CAD build for the part. Positions are in the model's coordinates, mm. A direction names the side the tool comes from. Give positions to 0.01 mm unless a question says otherwise; leave off trailing zeros. Order: outer loops, then holes, each group sorted by start corner. A loop starts at its lowest first (then second) coordinate and runs counter-clockwise, first axis right, second up. Notation, with made-up numbers: (5.5, 7.25) -> (32.5, 7.25) arc R15 ccw to (32.5, 36.25) -> close; hole circle Ø11 at (57, -15). An arc over 180 degrees is marked (long way). Use one line per item in the form item = value. Start each with the question number.
1) Tool access for faces 4 (the face through (0, 0, -6)), 5 (the face through (0.86, 0.51, 1.06)): list every direction of +Z, -Z, +X, -X, +Y, -Y with a clear straight run to the whole face (end or side of a thin tool).
2) Probe line 1 (Y direction, x = -0.55, z = 1.25); line 2 (Y direction, x = 0.4, z = 0.5); line 3 (Y direction, x = -0.2, z = -5.5). List the from-to ranges inside material, lowest first.
3) Cut at A-A, the plane z = -1. Give the cut face in (x, y), and give its area (3 significant figures).
4) Drop flat-ended pins along their axis: P1, Ø0.5, axis at x = 0, z = 1, coming from the -Y side; P2, Ø3, axis at y = -1.5, z = -3, coming from the +X side; P3, Ø3, axis at y = -1.5, z = -3, coming from the -X side. Give the stop position or say it passes through.
5) Mould opens along X. For faces 1 (the face through (0.1, 0, 0)), 2 (the face through (0, 2, 0)), 3 (the face through (-1.5, 0.07, -2.87)) say: pulls with the +X half, pulls with the -X half, needs draft (parallel to the pull), parting line crosses it, or undercut.
Solid Edge part; units mm, degrees
sketch "Sketch1" plane through (0, 0, 0) normal (0, -1, 0) x (1, 0, 0)
  line L0 (0, -6) -> (1.5, -6)
  line L1 (1.5, -6) -> (1.5, -0.115)
  arc A0 (1.5, -0.105) -> (1.5, -0.115) centre (1.5038, -0.11) ccw
  line L2 (1.5, -0.105) -> (1.5, 0)
  line L3 (1.5, 0) -> (2.85, 0)
  line L4 (2.85, 0) -> (2.85, 0.165)
  arc A1 (1.27, 1.65) -> (2.85, 0.165) centre (-0.3628, -1.6703) cw
  line L5 (0, 1.65) -> (1.27, 1.65)
  dimension "D1" = 1.5
revolve "RevolvedProtrusion1" add sketch "Sketch1" angle 360 about axis through (0, 0, 5) along (0, 0, -1)
sketch "Sketch2" plane through (0, 0, 0) normal (0, -1, 0) x (1, 0, 0)
  line L0 (0, -0.0566) -> (1.1545, 0.61)
  line L1 (1.1545, 0.61) -> (1.1545, 1.65)
  line L2 (1.1545, 1.65) -> (0, 1.65)
revolve "RevolvedCutout1" cut sketch "Sketch2" angle 360 about axis through (0, 0, 5.3) along (0, 0, -1)
sketch "Sketch3" plane through (0, 0, 0) normal (0, 0, -1) x (0, 1, 0)
  arc A0 (-1, 0.577) -> (-1, -0.577) centre (0, 0) ccw
  line L0 (-1, 0.577) -> (-1, -0.577)
extrude "Protrusion1" add sketch "Sketch3" against normal blind 1.65
pattern_circular "Pattern1" count 6 over 360 about axis through (0, 0, 0) along (0, 0, -1) of "Protrusion1"
fillet "Round_1" radius 0.185 1 edges at (-1.27, 0, 1.65)
sketch "Sketch4" plane through (0, 0, 0) normal (0, -1, 0) x (1, 0, 0)
  line L0 (0, 0.9501) -> (1.2122, 1.65)
  line L1 (1.2122, 1.65) -> (0, 1.65)
revolve "RevolvedCutout2" cut sketch "Sketch4" angle 360 about axis through (0, 0, 5.3) along (0, 0, -1)
sketch "Sketch5" plane through (0, 0, 0) normal (0, -1, 0) x (1, 0, 0)
  line L0 (-1.5, 0) -> (-1.5, -0.1)
  line L1 (-1.6, 0) -> (-1.5, 0)
  arc A0 (-1.6, 0) -> (-1.5, -0.1) centre (-1.6, -0.1) cw
revolve "RevolvedProtrusion2" add sketch "Sketch5" angle 360 about axis through (0, 0, -0.5) along (0, 0, 1)
cosmetic_thread "Thread1"
chamfer "Chamfer1" distance 0.3065 angle 45 1 edges at (-1.5, 0, -6)
properties material "Stahl"
Result:
q1.face_4 = -Z, +X, -X, +Y, -Y
q1.face_5 = +Z
q2.line_1 = -1.83 to -1, 1 to 1.83
q2.line_2 = -2.6 to -0.88, 0.88 to 2.6
q2.line_3 = -1.49 to 1.49
q3.outline = circle Ø3 at (0, 0)
q3.area = 7.07 mm²
q4.P1 = -2.44
q4.P2 = 1.5
q4.P3 = -1.5
q5.face_1 = undercut
q5.face_2 = needs draft
q5.face_3 = parting line crosses it
